Can you work these out from the drawing? Everything is in mm from the part's minimum corner. Give positions to 0.01 mm unless a question says otherwise; leave off trailing zeros. Order: outer loops, then holes, each group sorted by start corner. A loop starts at its lowest first (then second) coordinate and runs counter-clockwise, first axis right, second up. Notation, with made-up numbers: M 1.25,45.5 L 47.25,45.5 A10 cw 47.25,58.5 Z; hole C -26.75,54.25 d9. An arc over 180 degrees is marked long. Answer as a JSON object with one key per item and string values.
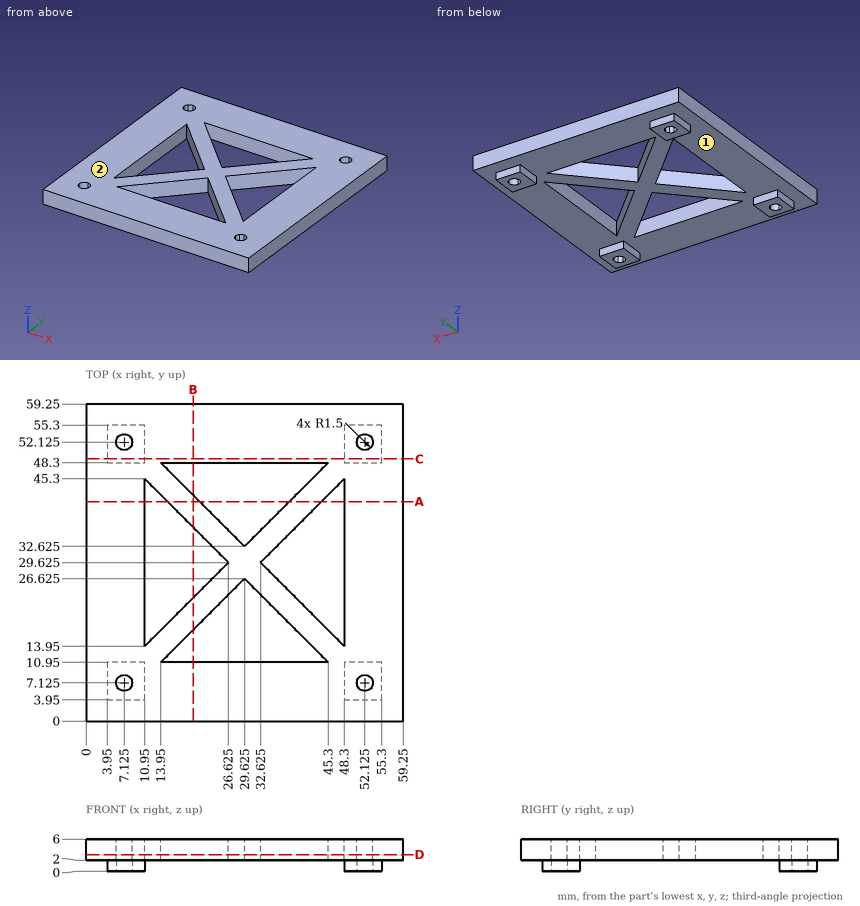
1) I want a section at C-C on y = 49. Write out the boundary of the cut face in (x, z), and give its area (3 significant figures).
Results found:
{"outline": "M 0,2 L 3.95,2 L 3.95,0 L 10.95,0 L 10.95,2 L 48.3,2 L 48.3,0 L 55.3,0 L 55.3,2 L 59.25,2 L 59.25,6 L 0,6 Z", "area": "265 mm²"}
2) I need wall thicknesses on L1, parallel to Y at x = 52, z = 1.1; L2, parallel to X at y = 18.5, z = 2.3; L3, parallel to Y at x = 52.5, z = 2.6. Which ranges of each line are inside material? Lowest first, please.
Results found:
{"L1": "y = 3.95 to 5.63, 8.62 to 10.95, 48.3 to 50.63, 53.62 to 55.3", "L2": "x = 0 to 10.95, 15.5 to 21.5, 37.75 to 43.75, 48.3 to 59.25", "L3": "y = 0 to 5.67, 8.58 to 50.67, 53.58 to 59.25"}
3) Thinking about a two-plate mould opening in X: for the marked faces 1 and 2, which applies, pulls with the +X half, pulls with the -X half, needs draft (parallel to the pull), parting line crosses it, or undercut?
Results found:
{"face 1": "undercut", "face 2": "needs draft"}
4) I want a section at D-D on z = 3.1. Count the separate pieces of the cut face and the enclosed holes in it, and give its area (3 significant figures).
Results found:
{"separate pieces": "1", "enclosed holes": "8", "area": "2,500 mm²"}
5) I'm going to push flat-ended pins straight in: pin 1 Ø1 at (x, z) = (6.5, 1) entering from +Y; pin 2 Ø0.6 at (y, z) = (53.5, 1) entering from +X; pin 3 Ø1 at (y, z) = (50.5, 1) entering from -X; pin 4 Ø6 at (x, y) = (45, 31) entering from +Z. Where does each tip first touch, or does it pass through?
Results found:
{"pin 1": "stops at y = 55.3", "pin 2": "stops at x = 55.3", "pin 3": "stops at x = 3.95", "pin 4": "passes through"}
6) I want a section at A-A on y = 41. Write out the boundary of the cut face in (x, z), and give its area (3 significant figures).
Results found:
{"outline": "M 0,2 L 10.95,2 L 10.95,6 L 0,6 Z; M 15.25,2 L 21.25,2 L 21.25,6 L 15.25,6 Z; M 38,2 L 44,2 L 44,6 L 38,6 Z; M 48.3,2 L 59.25,2 L 59.25,6 L 48.3,6 Z", "area": "136 mm²"}
7) I want a section at B-B on x = 20. Write out the boundary of the cut face in (y, z), and give its area (3 significant figures).
Results found:
{"outline": "M 0,2 L 10.95,2 L 10.95,6 L 0,6 Z; M 17,2 L 23,2 L 23,6 L 17,6 Z; M 36.25,2 L 42.25,2 L 42.25,6 L 36.25,6 Z; M 48.3,2 L 59.25,2 L 59.25,6 L 48.3,6 Z", "area": "136 mm²"}
